Verification items for the finished model (mm, model axes). Face numbers are marked on the shaded views. A direction names the side the tool comes from. Round coordinates to 2 decimals unless told otherwise and drop trailing zeros. Write each loop counter-clockwise with the first axis right and the second up, starting at its lowest first coordinate (ties: lowest second). Pieces come first, ordered by that corner, then holes. Notation, with made-up numbers: (79, 79) - (133, 79) arc R30 ccw to (133, 111) - close; hole circle Ø5 at (29, 57). An arc over 180 degrees is marked (long way). Answer as a JSON object with one key per item and string values. Group by question number.
1) Set-up check for the marked faces 1, 2 and 3: record each of +Z, -Z, +X, -X, +Y, -Y from which the full face is reachable in a straight line by a thin tool's end or side.
2) Section check C-C (x = 8). Enter the section's corners in (y, z), then the cut area to 3 significant figures.
3) Section check D-D (z = -40). Enter the section's corners in (x, y) (3 decimals), then the cut area to 3 significant figures.
4) Mould release check, pull along X, two halves, no side actions. Record for the marked faces 4 and 5: +X half, -X half, draft (parallel to the pull), parting line (faces both ways), or undercut.
5) Section check B-B (x = 0). Enter the section's corners in (y, z) (1 decimal), then the cut area to 3 significant figures.
6) Thickness scan on line 1 (Z direction, x = 0, y = 1.7) (3 decimals); line 2 (Z direction, x = 3.5, y = 3.5); line 3 (Z direction, x = -6.5, y = 4.25). Record the ranges inside material, lowest first.
7) Section check A-A (z = -25). Enter the section's corners in (x, y) (3 decimals).
8) Go/stop test with flat-tipped pins: pin 1 Ø4 at (x, z) = (1, -29) entering from +Y; pin 2 Ø6 at (x, z) = (0, -25) entering from +Y; pin 3 Ø4 at (x, y) = (-3, 2) entering from +Z; pin 4 Ø0.6 at (y, z) = (9, -50.5) entering from +X. Record where each tip stops, or that it passes through.
```python
from build123d import *

# Parameters (mm, degrees)
BOSS_EXTRUDE1_DEPTH = 75
SKETCH3_R           = 5.155
CUT_EXTRUDE2_DEPTH  = 6.73
SKETCH4_R           = 3.365
CUT_EXTRUDE3_DEPTH  = 2.54
SKETCH5_R           = 1.5
CUT_EXTRUDE4_DEPTH  = 3
SKETCH6_R           = 1.5
BOSS_EXTRUDE2_DEPTH = 3


with BuildPart() as part:
    # Sketch1 → Boss-Extrude1 (new body)
    with BuildSketch(Plane.XY):
        Polygon((6.3246, 9.017), (6.3246, 9.271), (9.1186, 9.271), (9.1186, 8.509), (5.926144338, 2.921), (9.525, 2.921), (9.525, -0.254), (6.3246, -0.254), (6.3246, 0), (-6.3246, 0), (-6.3246, -0.254), (-9.525, -0.254), (-9.525, 2.921), (-5.926144338, 2.921), (-9.1186, 8.509), (-9.1186, 9.271), (-6.3246, 9.271), (-6.3246, 9.017), align=None)
    extrude(amount=-BOSS_EXTRUDE1_DEPTH)

    # Sketch3 → Cut-Extrude2 (cut)
    with BuildSketch(Plane(origin=(0, 9.017, 0), x_dir=(1, 0, 0), z_dir=(0, 1, 0))):
        with Locations(Location((0, 25, 0), (0, 0, 180))):
            Circle(SKETCH3_R)
        with Locations(Location((0, 50, 0), (0, 0, 180))):
            Circle(SKETCH3_R)
    extrude(amount=-CUT_EXTRUDE2_DEPTH, mode=Mode.SUBTRACT)

    # Sketch4 → Cut-Extrude3 (cut)
    with BuildSketch(Plane.XZ):
        with Locations((0, -25)):
            Circle(SKETCH4_R)
        with Locations((0, -50)):
            Circle(SKETCH4_R)
    extrude(amount=-CUT_EXTRUDE3_DEPTH, mode=Mode.SUBTRACT)

    # Sketch5 → Cut-Extrude4 (cut)
    with BuildSketch(Plane(origin=(0, 0, -75), x_dir=(-1, 0, 0), z_dir=(0, 0, -1))):
        with Locations((0, 4.5085)):
            Circle(SKETCH5_R)
    extrude(amount=-CUT_EXTRUDE4_DEPTH, mode=Mode.SUBTRACT)

    # Sketch6 → Boss-Extrude2 (add)
    with BuildSketch(Plane.XY):
        with Locations(Location((0, 4.5085, 0), (0, 0, 180))):
            Circle(SKETCH6_R)
    extrude(amount=BOSS_EXTRUDE2_DEPTH)


solid = part.part
```
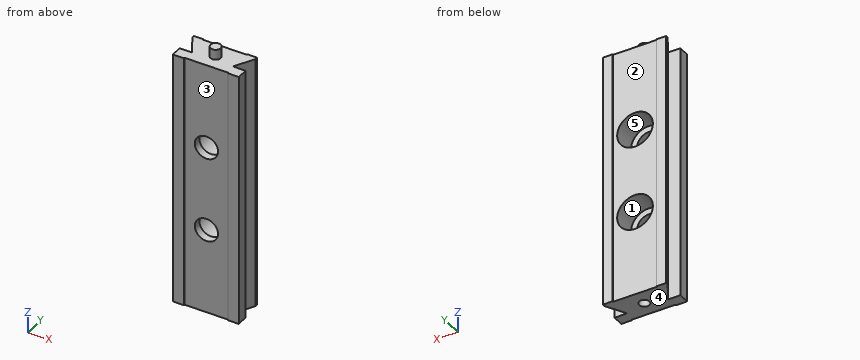
Returned:
{
 "1": {"face 1": "+Y", "face 2": "+Z, -Z, +Y", "face 3": "+Z, -Z, -Y"},
 "2": {"outline": "(-0.25, -75) - (2.92, -75) - (2.92, 0) - (-0.25, 0) - close; (6.55, -75) - (9.27, -75) - (9.27, 0) - (6.55, 0) - close", "area": "442 mm2"},
 "3": {"outline": "(-9.525, -0.254) - (-6.325, -0.254) - (-6.325, 0) - (6.325, 0) - (6.325, -0.254) - (9.525, -0.254) - (9.525, 2.921) - (5.926, 2.921) - (9.119, 8.509) - (9.119, 9.271) - (6.325, 9.271) - (6.325, 9.017) - (-6.325, 9.017) - (-6.325, 9.271) - (-9.119, 9.271) - (-9.119, 8.509) - (-5.926, 2.921) - (-9.525, 2.921) - close", "area": "152 mm2"},
 "4": {"face 4": "draft", "face 5": "undercut"},
 "5": {"outline": "(0, -75) - (3, -75) - (3, -72) - (6, -72) - (6, -75) - (9, -75) - (9, -55.2) - (2.3, -55.2) - (2.3, -53.4) - (0, -53.4) - close; (0, -46.6) - (2.3, -46.6) - (2.3, -44.8) - (9, -44.8) - (9, -30.2) - (2.3, -30.2) - (2.3, -28.4) - (0, -28.4) - close; (0, -21.6) - (2.3, -21.6) - (2.3, -19.8) - (9, -19.8) - (9, 0) - (6, 0) - (6, 3) - (3, 3) - (3, 0) - (0, 0) - close", "area": "507 mm2"},
 "6": {"line 1": "-75 to -53.365, -46.635 to -28.365, -21.635 to 0", "line 2": "-75 to -53.78, -46.22 to -28.78, -21.22 to 0", "line 3": "-75 to 0"},
 "7": {"outline": "(-9.525, -0.254) - (-6.325, -0.254) - (-6.325, 0) - (-3.365, 0) - (-3.365, 2.287) - (-5.155, 2.287) - (-5.155, 9.017) - (-6.325, 9.017) - (-6.325, 9.271) - (-9.119, 9.271) - (-9.119, 8.509) - (-5.926, 2.921) - (-9.525, 2.921) - close; (3.365, 0) - (6.325, 0) - (6.325, -0.254) - (9.525, -0.254) - (9.525, 2.921) - (5.926, 2.921) - (9.119, 8.509) - (9.119, 9.271) - (6.325, 9.271) - (6.325, 9.017) - (5.155, 9.017) - (5.155, 2.287) - (3.365, 2.287) - close"},
 "8": {"pin 1": "y = 9.02", "pin 2": "through", "pin 3": "z = 0", "pin 4": "x = 9.12"}
}
